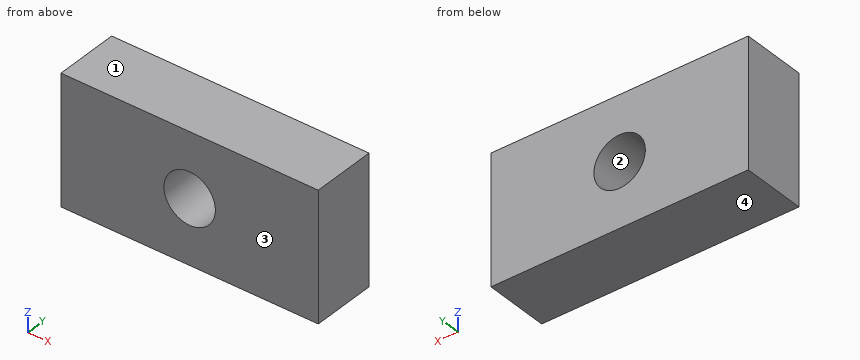
from build123d import *

# Parameters (mm, degrees)
SKETCH2_W           = 40
SKETCH2_H           = 20
BOSS_EXTRUDE1_DEPTH = 10
CUT_EXTRUDE1_REACH  = 52.396
SKETCH3_R           = 4


with BuildPart() as part:
    # Sketch2 → Boss-Extrude1 (new body)
    with BuildSketch(Plane(origin=(0, 0, 0), x_dir=(1, 0, 0), z_dir=(0, 1, 0))):
        with Locations((-16.330703266, -23.463822806)):
            Rectangle(SKETCH2_W, SKETCH2_H)
    extrude(amount=BOSS_EXTRUDE1_DEPTH)

    # Sketch3 → Cut-Extrude1 (cut, up to next)
    with BuildSketch(Plane(origin=(0, 10, 0), x_dir=(1, 0, 0), z_dir=(0, 1, 0)), mode=Mode.PRIVATE) as cut_extrude1_sk1:
        with Locations(Location((-16.330703266, -23.463822806, 0), (0, 0, 270))):
            Circle(SKETCH3_R)
    cut_extrude1_tool1 = extrude(cut_extrude1_sk1.sketch, amount=-CUT_EXTRUDE1_REACH, mode=Mode.PRIVATE) & part.part
    add(cut_extrude1_tool1.solids().sort_by_distance((-16.330703, 10, 23.463823))[0], mode=Mode.SUBTRACT)


solid = part.part
Could you check a few things on this model? Use its own coordinates, in mm. Face numbers are marked on the shaded views. Coordinates: 2 decimals unless noted, no trailing zeros. Order: outer loops, then holes, each group sorted by start corner. A loop starts at its lowest first (then second) coordinate and runs counter-clockwise, first axis right, second up.
Q1. Thinking about a two-plate mould opening in Z: for the marked faces 1, 2, 3 and 4, which applies, released by +Z, released by -Z, zero draft, split by the parting line, or undercut?
Q2. Suppose I cut it at A-A on z = 22. Please give me the cut outline in (x, y).
Q3. Suppose I cut it at C-C on y = 5.5. Please give me the cut outline in (x, z).
Q4. Suppose I cut it at B-B on x = -18. Please give me the cut outline in (y, z).
Q5. Please list where these lines run through material, in increasing order: L1, parallel to X at y = 0.75, z = 21.5; L2, parallel to Z at x = -19, y = 6.75; L3, parallel to X at y = 6.75, z = 22.
Answer:
1. face 1: released by +Z
1. face 2: undercut
1. face 3: zero draft
1. face 4: released by -Z
2. outline: (-36.33, 0) - (-20.05, 0) - (-20.05, 10) - (-36.33, 10) - close; (-12.61, 0) - (3.67, 0) - (3.67, 10) - (-12.61, 10) - close
3. outline: (-36.33, 13.46) - (3.67, 13.46) - (3.67, 33.46) - (-36.33, 33.46) - close; hole circle Ø8 at (-16.33, 23.46)
4. outline: (0, 13.46) - (10, 13.46) - (10, 19.83) - (0, 19.83) - close; (0, 27.1) - (10, 27.1) - (10, 33.46) - (0, 33.46) - close
5. L1: x = -36.33 to -19.82, -12.85 to 3.67
5. L2: z = 13.46 to 20.48, 26.44 to 33.46
5. L3: x = -36.33 to -20.05, -12.61 to 3.67
